Design review of the part built by this model. Coordinates are the model's own, in mm. Give positions to 0.01 mm unless a question says otherwise; leave off trailing zeros. Loops run counter-clockwise (first coordinate to the right, second up) from the corner with the lowest first, then second, coordinate; pieces in that order, holes last.
from build123d import *

# Parameters (mm, degrees)
SKETCH1_W               = 190.5
SKETCH1_H               = 241.3
BOSS_EXTRUDE1_DEPTH     = 2.54
FILLET1_R               = 5.08
CUT_EXTRUDE1_DEPTH      = 154.738208003
CUT_EXTRUDE1_DEPTH_BACK = 154.738208003
SKETCH2_R               = 3.175


with BuildPart() as part:
    # Sketch1 → Boss-Extrude1 (new body)
    with BuildSketch(Plane.YZ):
        Rectangle(SKETCH1_W, SKETCH1_H)
    extrude(amount=BOSS_EXTRUDE1_DEPTH)

    # Fillet1
    fillet1_edges = [part.edges().sort_by_distance(p)[0] for p in [
        (1.27, 95.25, -120.65),
        (1.27, -95.25, -120.65),
        (1.27, -95.25, 120.65),
        (1.27, 95.25, 120.65),
    ]]
    fillet(fillet1_edges, radius=FILLET1_R)

    # Sketch2 → Cut-Extrude1 (cut, two sides: drawn at the far end of the back side and taken through both)
    with BuildSketch(Plane(origin=(2.54, 0, 0), x_dir=(0, 0, -1), z_dir=(1, 0, 0)).offset(-CUT_EXTRUDE1_DEPTH_BACK)):
        with Locations((-574.675, 0)):
            Circle(SKETCH2_R)
        with Locations((-725.4875, 79.375)):
            Circle(SKETCH2_R)
        with Locations((-831.85, 79.375)):
            Circle(SKETCH2_R)
        with Locations((-938.2125, 79.375)):
            Circle(SKETCH2_R)
        with Locations((-1044.575, 79.375)):
            Circle(SKETCH2_R)
        with Locations((-1044.575, -79.375)):
            Circle(SKETCH2_R)
        with Locations((-1044.575, 0)):
            Circle(SKETCH2_R)
        with Locations((-574.675, 79.375)):
            Circle(SKETCH2_R)
        with Locations((-468.3125, 79.375)):
            Circle(SKETCH2_R)
        with Locations((-574.675, -79.375)):
            Circle(SKETCH2_R)
        with Locations((-725.4875, -79.375)):
            Circle(SKETCH2_R)
        with Locations((-619.125, -79.375)):
            Circle(SKETCH2_R)
        with Locations((-619.125, 0)):
            Circle(SKETCH2_R)
        with Locations((-619.125, 79.375)):
            Circle(SKETCH2_R)
        with Locations((-255.5875, 79.375)):
            Circle(SKETCH2_R)
        with Locations((-361.95, 79.375)):
            Circle(SKETCH2_R)
        with Locations((-938.2125, -79.375)):
            Circle(SKETCH2_R)
        with Locations((-831.85, -79.375)):
            Circle(SKETCH2_R)
        with Locations((-149.225, -79.375)):
            Circle(SKETCH2_R)
        with Locations((-255.5875, -79.375)):
            Circle(SKETCH2_R)
        with Locations((-149.225, 79.375)):
            Circle(SKETCH2_R)
        with Locations((-361.95, -79.375)):
            Circle(SKETCH2_R)
        with Locations((-149.225, 0)):
            Circle(SKETCH2_R)
        with Locations((-468.3125, -79.375)):
            Circle(SKETCH2_R)
        with Locations((0, 79.375)):
            Circle(SKETCH2_R)
        with Locations((0, -79.375)):
            Circle(SKETCH2_R)
        with Locations((-104.775, -79.375)):
            Circle(SKETCH2_R)
        with Locations((-104.775, 79.375)):
            Circle(SKETCH2_R)
        with Locations((104.775, 0)):
            Circle(SKETCH2_R)
        with Locations((-104.775, 0)):
            Circle(SKETCH2_R)
        with Locations((104.775, -79.375)):
            Circle(SKETCH2_R)
        with Locations((104.775, 79.375)):
            Circle(SKETCH2_R)
    extrude(amount=CUT_EXTRUDE1_DEPTH + CUT_EXTRUDE1_DEPTH_BACK, mode=Mode.SUBTRACT)


solid = part.part
Q1. Insertion check: pin 1 (4 mm diameter, centred on y = 79.375, z = -104.775, fed in from +X); pin 2 (10 mm diameter, centred on y = 79.375, z = 104.775, fed in from -X). Each pin has a flat end and moves straight along its axis. Give the tip position at first contact, or say it passes through.
Results:
pin 1: passes through
pin 2: stops at x = 0
Q2. Take a section at A-A (y = 0). Give the boundary of the cut face in (x, z).
Results:
outline: (0, -120.65) - (2.54, -120.65) - (2.54, -107.95) - (0, -107.95) - close; (0, -101.6) - (2.54, -101.6) - (2.54, 101.6) - (0, 101.6) - close; (0, 107.95) - (2.54, 107.95) - (2.54, 120.65) - (0, 120.65) - close
Q3. Draft analysis for pull direction Y (two halves, no side actions). For faces 1 (the face through (1.252, -76.227, 105.188)), 2 (the face through (1.288, -93.801, -119.122)), 3 (the face through (0, -1, 2)), 4 (the face through (1.288, 93.722, -119.201)), state which applies: pulls with the +Y half, pulls with the -Y half, needs draft (parallel to the pull), parting line crosses it, or undercut.
Results:
face 1: undercut
face 2: pulls with the -Y half
face 3: needs draft
face 4: pulls with the +Y half
Q4. Take a section at B-B (z = 0). Give the boundary of the cut face in (x, y), plus the area to 3 significant figures.
Results:
outline: (0, -95.25) - (2.54, -95.25) - (2.54, -82.55) - (0, -82.55) - close; (0, -76.2) - (2.54, -76.2) - (2.54, 76.2) - (0, 76.2) - close; (0, 82.55) - (2.54, 82.55) - (2.54, 95.25) - (0, 95.25) - close
area: 452 mm2
Q5. Take a section at C-C (z = -105). Give the boundary of the cut face in (x, y).
Results:
outline: (0, -95.25) - (2.54, -95.25) - (2.54, -82.54) - (0, -82.54) - close; (0, -76.21) - (2.54, -76.21) - (2.54, -3.17) - (0, -3.17) - close; (0, 3.17) - (2.54, 3.17) - (2.54, 76.21) - (0, 76.21) - close; (0, 82.54) - (2.54, 82.54) - (2.54, 95.25) - (0, 95.25) - close
Q6. Wall thickness on line 1 (Y direction, x = 1.8, z = 0); line 2 (Z direction, x = 2, y = 0); line 3 (Y direction, x = 0.4, z = 104): over which ranges is each line inside the solid? List them lowest first.
Results:
line 1: y = -95.25 to -82.55, -76.2 to 76.2, 82.55 to 95.25
line 2: z = -120.65 to -107.95, -101.6 to 101.6, 107.95 to 120.65
line 3: y = -95.25 to -82.45, -76.3 to -3.08, 3.08 to 76.3, 82.45 to 95.25
